Drawing for the job (mm, zero at the part's lowest x, y, z). A direction names the side the tool comes from. Round coordinates to 2 decimals unless told otherwise and drop trailing zeros. Write each loop counter-clockwise with the first axis right and the second up, starting at its lowest first coordinate (ties: lowest second). Pieces come first, ordered by that corner, then holes. Notation, with made-up numbers: (-21.75, 8) -> (16.25, 8) arc R22 ccw to (16.25, 30) -> close; hole circle Ø5 at (0.25, 10). An arc over 180 degrees is marked (long way). One line per question, with ' | ' between items.
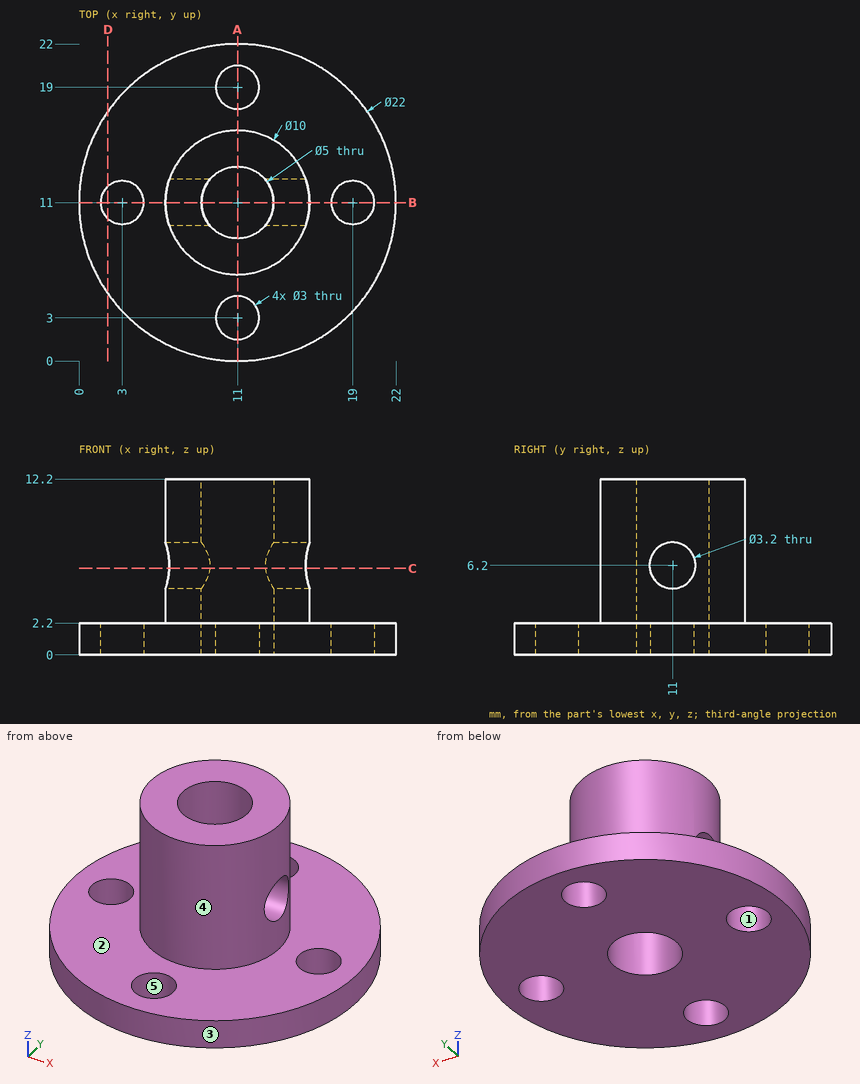
(1) Slice it at B-B (y = 11). Write the cut outline in (x, z), then the cut area to 3 significant figures.
Calculated:
outline: (0, 0) -> (1.5, 0) -> (1.5, 2.2) -> (0, 2.2) -> close; (4.5, 0) -> (8.5, 0) -> (8.5, 4.6) -> (6, 4.6) -> (6, 2.2) -> (4.5, 2.2) -> close; (6, 7.8) -> (8.5, 7.8) -> (8.5, 12.2) -> (6, 12.2) -> close; (13.5, 0) -> (17.5, 0) -> (17.5, 2.2) -> (16, 2.2) -> (16, 4.6) -> (13.5, 4.6) -> close; (13.5, 7.8) -> (16, 7.8) -> (16, 12.2) -> (13.5, 12.2) -> close; (20.5, 0) -> (22, 0) -> (22, 2.2) -> (20.5, 2.2) -> close | area: 58.2 mm2
(2) Slice it at C-C (z = 6). Write the cut outline in (x, y).
Calculated:
outline: (6.26, 9.41) arc R5 ccw to (15.74, 9.41) -> (12.93, 9.41) arc R2.5 cw to (9.07, 9.41) -> close; (6.26, 12.59) -> (9.07, 12.59) arc R2.5 cw to (12.93, 12.59) -> (15.74, 12.59) arc R5 ccw to start
(3) Slice it at A-A (x = 11). Write the cut outline in (y, z), then the cut area to 3 significant figures.
Calculated:
outline: (0, 0) -> (1.5, 0) -> (1.5, 2.2) -> (0, 2.2) -> close; (4.5, 0) -> (8.5, 0) -> (8.5, 12.2) -> (6, 12.2) -> (6, 2.2) -> (4.5, 2.2) -> close; (13.5, 0) -> (17.5, 0) -> (17.5, 2.2) -> (16, 2.2) -> (16, 12.2) -> (13.5, 12.2) -> close; (20.5, 0) -> (22, 0) -> (22, 2.2) -> (20.5, 2.2) -> close | area: 74.2 mm2
(4) Drop flat-ended pins along their axis: pin 1 (10 mm diameter, centred on x = 7.5, y = 19.5, fed in from +Z); pin 2 (5 mm diameter, centred on x = 11, y = 3, fed in from +Z); pin 3 (2.5 mm diameter, centred on y = 11, z = 6.2, fed in from -X); pin 4 (3.5 mm diameter, centred on y = 11, z = 6.2, fed in from -X). Give the stop position or say it passes through.
Calculated:
pin 1: z = 12.2 | pin 2: z = 2.2 | pin 3: through | pin 4: x = 6
(5) Slice it at D-D (x = 2). Write the cut outline in (y, z), then the cut area to 3 significant figures.
Calculated:
outline: (4.68, 0) -> (9.88, 0) -> (9.88, 2.2) -> (4.68, 2.2) -> close; (12.12, 0) -> (17.32, 0) -> (17.32, 2.2) -> (12.12, 2.2) -> close | area: 22.9 mm2
(6) Mould opens along Y. For the marked faces 1, 2 and 3 say: pulls with the +Y half, pulls with the -Y half, needs draft (parallel to the pull), parting line crosses it, or undercut.
Calculated:
face 1: undercut | face 2: needs draft | face 3: parting line crosses it
(7) 3-axis set-ups, long thin cutter, end or side, ignore diameter. For the marked faces 4 and 5: which of +Z, -Z, +X, -X, +Y, -Y reach the whole face in a straight line?
Calculated:
face 4: +Z | face 5: +Z, -Z
(8) Wall check: line 1 (X direction, y = 11, z = 3.5); line 2 (Y direction, x = 18.25, z = 0.5); line 3 (Z direction, x = 1.75, y = 16.25). Give the ranges that are in metal, low to high. Write a range as from..to.
Calculated:
line 1: 6..8.5, 13.5..16 | line 2: 2.73..9.7, 12.3..19.27 | line 3: 0..2.2
